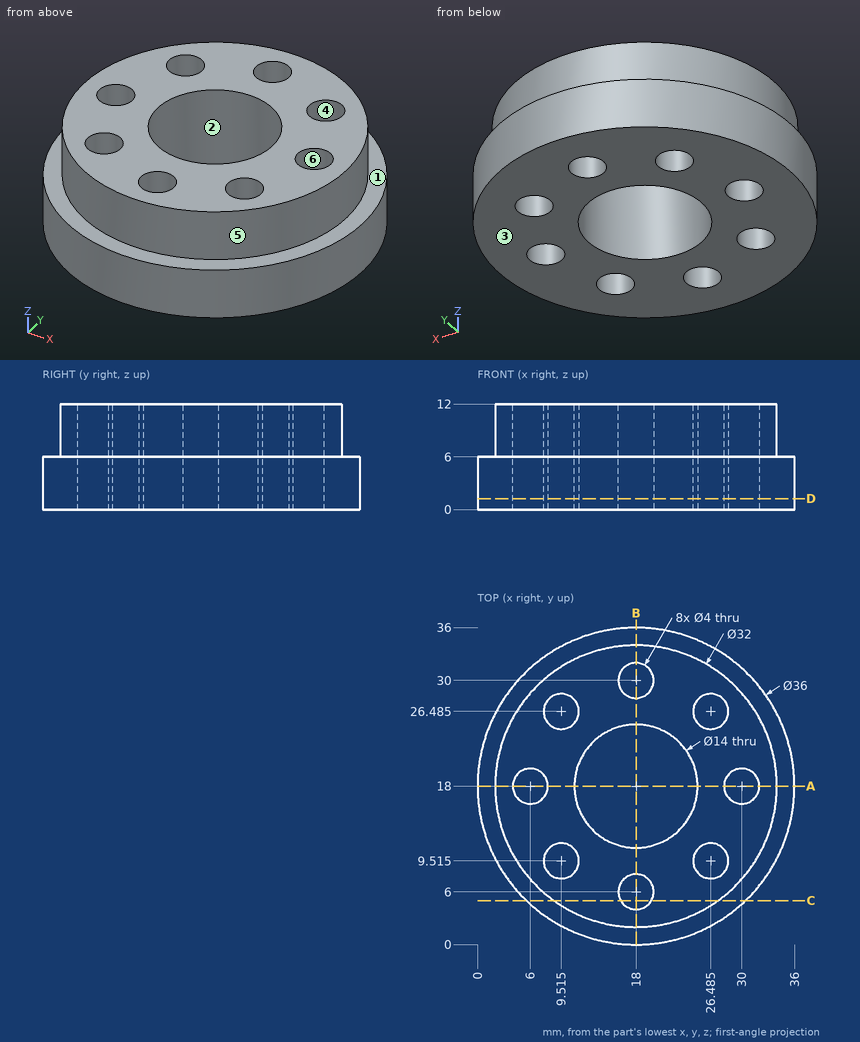
Answer from the drawing. Dimensions are ordinates in mm from the lowest x, y and z of the part. A direction names the side the tool comes from. Give positions to 0.01 mm unless a question says otherwise; leave off trailing zeros. Write each loop counter-clockwise with the first axis right and the second up, starting at its lowest first coordinate (ties: lowest second). Pieces come first, ordered by that corner, then holes. Notation, with made-up numbers: (57.5, 47.5) -> (69.5, 47.5) arc R34 ccw to (69.5, 85.5) -> close; hole circle Ø11 at (-36.75, -37). An arc over 180 degrees is marked (long way). One line per question, with ' | ' between items. Start each with the question number.
1. Find the intervals of material crossed by probe 1 along X at (y, z) = (10.5, 8.5) (1 decimal); probe 2 along X at (y, z) = (27.5, 3.5); probe 3 along Y at (x, z) = (17, 1), in increasing order.
2. Given pin 1 Ø2.5 at (x, y) = (26.49, 26.49) entering from +Z; pin 2 Ø2 at (x, y) = (32, 29) entering from +Z; pin 3 Ø1.5 at (y, z) = (4, 9) entering from +X; pin 4 Ø3 at (x, z) = (5.5, 7) entering from +Y (1 decimal), each flat-ended and moving along its own axis, determine where each tip first touches the part or whether it passes through.
3. Section C-C (y = 5) is taken. Determine the outline of the cut face in (x, z).
4. Section A-A (y = 18) is taken. Determine the outline of the cut face in (x, z), plus the area to 3 significant figures.
5. Section D-D (z = 1.25) is taken. State how many separate pieces and enclosed holes the cut face has.
6. For a pull along Y with two mould halves and no side action, classify the marked faces 3, 4, 5 and 6 as pulls with the +Y half, pulls with the -Y half, needs draft (parallel to the pull), parting line crosses it, or undercut.
7. For the marked faces 1 and 2, determine the directions among +Z, -Z, +X, -X, +Y, -Y from which every point of the face is accessible in a straight line to the end or side of a thin tool.
Response values:
1) probe 1: 3.9 to 7.8, 11.3 to 24.7, 28.2 to 32.1 | probe 2: 2.71 to 7.79, 11.24 to 24.76, 28.21 to 33.29 | probe 3: 0.03 to 4.27, 7.73 to 11.07, 24.93 to 28.27, 31.73 to 35.97
2) pin 1: through | pin 2: z = 6 | pin 3: x = 26.97 | pin 4: y = 31.9
3) outline: (5.55, 0) -> (16.27, 0) -> (16.27, 12) -> (8.67, 12) -> (8.67, 6) -> (5.55, 6) -> close; (19.73, 0) -> (30.45, 0) -> (30.45, 6) -> (27.33, 6) -> (27.33, 12) -> (19.73, 12) -> close
4) outline: (0, 0) -> (4, 0) -> (4, 12) -> (2, 12) -> (2, 6) -> (0, 6) -> close; (8, 0) -> (11, 0) -> (11, 12) -> (8, 12) -> close; (25, 0) -> (28, 0) -> (28, 12) -> (25, 12) -> close; (32, 0) -> (36, 0) -> (36, 6) -> (34, 6) -> (34, 12) -> (32, 12) -> close | area: 144 mm2
5) separate pieces: 1 | enclosed holes: 9
6) face 3: needs draft | face 4: undercut | face 5: parting line crosses it | face 6: undercut
7) face 1: +Z | face 2: +Z, -Z
